from build123d import *

# Parameters (mm, degrees)
SKETCH1_R           = 6
BOSS_EXTRUDE1_DEPTH = 10
SKETCH2_R           = 1.025
CUT_EXTRUDE1_DEPTH  = 7
SKETCH4_R           = 2.1
CUT_EXTRUDE4_DEPTH  = 11.0000001
SKETCH5_W           = 0.95
SKETCH5_H           = 7.069146706
BOSS_EXTRUDE2_DEPTH = 1.2
SKETCH7_R           = 6
BOSS_EXTRUDE3_DEPTH = 1
SKETCH8_R           = 2.625
SKETCH8_W           = 2.25
SKETCH8_H           = 1.25
BOSS_EXTRUDE4_DEPTH = 6.5
SKETCH9_R           = 1.075
CUT_EXTRUDE5_DEPTH  = 6
CUT_EXTRUDE2_START  = -3
CUT_EXTRUDE2_DEPTH  = 1.85


with BuildPart() as part:
    # Sketch1 → Boss-Extrude1 (new body)
    with BuildSketch(Plane(origin=(0, 0, 0), x_dir=(1, 0, 0), z_dir=(0, 1, 0))):
        Circle(SKETCH1_R)
    extrude(amount=BOSS_EXTRUDE1_DEPTH)

    # Sketch2 → Cut-Extrude1 (cut, through all)
    with BuildSketch(Plane.XY):
        with Locations((0, 7)):
            Circle(SKETCH2_R)
    extrude(amount=-CUT_EXTRUDE1_DEPTH, mode=Mode.SUBTRACT)

    # Sketch4 → Cut-Extrude4 (cut, through all)
    with BuildSketch(Plane(origin=(0, 0, 0), x_dir=(1, 0, 0), z_dir=(0, 1, 0))):
        Circle(SKETCH4_R)
    extrude(amount=CUT_EXTRUDE4_DEPTH, mode=Mode.SUBTRACT)

    # Sketch5 → Boss-Extrude2 (add)
    with BuildSketch(Plane(origin=(0, 10, 0), x_dir=(1, 0, 0), z_dir=(0, 1, 0))):
        Rectangle(SKETCH5_W, SKETCH5_H)
    extrude(amount=-BOSS_EXTRUDE2_DEPTH)

    # Sketch7 → Boss-Extrude3 (add)
    with BuildSketch(Plane(origin=(0, 10, 0), x_dir=(1, 0, 0), z_dir=(0, 1, 0))):
        Circle(SKETCH7_R)
    extrude(amount=BOSS_EXTRUDE3_DEPTH)

    # Sketch8 → Boss-Extrude4 (add)
    with BuildSketch(Plane(origin=(0, 11, 0), x_dir=(1, 0, 0), z_dir=(0, 1, 0))):
        Circle(SKETCH8_R)
        with Locations((0, -2.625)):
            Rectangle(SKETCH8_W, SKETCH8_H)
    extrude(amount=BOSS_EXTRUDE4_DEPTH)

    # Sketch9 → Cut-Extrude5 (cut)
    with BuildSketch(Plane(origin=(0, 17.5, 0), x_dir=(1, 0, 0), z_dir=(0, 1, 0))):
        Circle(SKETCH9_R)
    extrude(amount=-CUT_EXTRUDE5_DEPTH, mode=Mode.SUBTRACT)

    # Sketch3 → Cut-Extrude2 (cut)
    with BuildSketch(Plane.XY.offset(CUT_EXTRUDE2_START)):
        Polygon((0, 4.621316891), (2.06, 5.810658445), (2.06, 8.189341555), (2.06, 11.363105915), (-2.06, 11.363105915), (-2.06, 8.189341555), (-2.06, 5.810658445), align=None)
    extrude(amount=-CUT_EXTRUDE2_DEPTH, mode=Mode.SUBTRACT)


solid = part.part
CAD build for the part. Positions are in the model's coordinates, mm. A direction names the side the tool comes from. Coordinates: 2 decimals unless noted, no trailing zeros. Write each loop counter-clockwise with the first axis right and the second up, starting at its lowest first coordinate (ties: lowest second). Pieces come first, ordered by that corner, then holes. Notation, with made-up numbers: M 56,8 L 101,8 A19 ccw 101,18 Z; hole C -37.75,25 d8. An arc over 180 degrees is marked long. Answer as a JSON object with one key per item and string values. Group by question number.
1) Saw through at D-D (y = 14). Write the cut outline in (x, z) (3 decimals), plus the area to 3 significant figures.
2) Saw through at B-B (z = 0). Write the cut outline in (x, y) (3 decimals), plus the area to 3 significant figures.
3) Saw through at A-A (y = 9.75). Write the cut outline in (x, z) (3 decimals), plus the area to 3 significant figures.
4) Wall check: line 1 (Z direction, x = 0, y = 5); line 2 (Y direction, x = 0, z = -2.75) (3 decimals); line 3 (Z direction, x = 0, y = 3.75). Give the ranges that are in metal, low to high. Write a range as from..to.
5) Pin check, flat tips, straight feed: pin 1 Ø0.7 at (y, z) = (15.5, 3) entering from +X (3 decimals); pin 2 Ø1.8 at (x, y) = (0.5, 13) entering from +Z; pin 3 Ø0.6 at (y, z) = (7.5, -4) entering from -X. Stop position of each tip, or through.
6) Saw through at C-C (x = -0.25). Write the cut outline in (y, z), plus the area to 3 significant figures.
7) Tool access for faces 5 (the face through (-0.475, 9, 0)), 6 (the face through (-1.024, 7.045, -5.418)), 7 (the face through (2.06, 8, -4)), 8 (the face through (-1.301, 5.423, 5.857)): list every direction of +Z, -Z, +X, -X, +Y, -Y with a clear straight run to the whole face (end or side of a thin tool).
8) Mould opens along X. For faces 1 (the face through (-1, 5.2, -3.9)), 2 (the face through (1.125, 14, 3)), 3 (the face through (-1, 17.5, 1)), 4 (the face through (-1.125, 14, 3)) say: +X half, -X half, draft (parallel to the pull), parting line (faces both ways), or undercut.
Values follow:
{
 "1": {"outline": "M -1.125,2.372 A2.625 ccw long 1.125,2.372 L 1.125,3.25 L -1.125,3.25 Z; hole C 0,0 d2.15", "area": "19.6 mm2"},
 "2": {"outline": "M -6,0 L -2.1,0 L -2.1,10 L -0.475,10 L -0.475,8.8 L 0.475,8.8 L 0.475,10 L 2.1,10 L 2.1,0 L 6,0 L 6,11 L 2.625,11 L 2.625,17.5 L 1.075,17.5 L 1.075,11.5 L -1.075,11.5 L -1.075,17.5 L -2.625,17.5 L -2.625,11 L -6,11 Z", "area": "112 mm2"},
 "3": {"outline": "C 0,0 d12; hole M -2.06,-4.85 L 2.06,-4.85 L 2.06,-3 L -2.06,-3 Z; hole M -0.475,-2.046 L -0.475,2.046 A2.1 ccw Z; hole M 0.475,-2.046 A2.1 ccw 0.475,2.046 Z", "area": "95.6 mm2"},
 "4": {"line 1": "z = -6..-4.85, -3..-2.1, 2.1..6", "line 2": "y = 0..5.975, 8.025..11", "line 3": "z = -6..-2.1, 2.1..6"},
 "5": {"pin 1": "stops at x = 1.125", "pin 2": "stops at z = 3.25", "pin 3": "stops at x = -4.72"},
 "6": {"outline": "M 0,-5.99 L 6.01,-5.99 L 6.01,-4.85 L 4.77,-4.85 L 4.77,-3 L 6.01,-3 L 6.01,-2.09 L 0,-2.09 Z; M 0,2.09 L 8.8,2.09 L 8.8,-2.09 L 7.99,-2.09 L 7.99,-3 L 11,-3 L 11,-2.61 L 17.5,-2.61 L 17.5,-1.05 L 11.5,-1.05 L 11.5,1.05 L 17.5,1.05 L 17.5,3.25 L 11,3.25 L 11,5.99 L 0,5.99 Z; M 7.99,-5.99 L 11,-5.99 L 11,-4.85 L 7.99,-4.85 Z", "area": "105 mm2"},
 "7": {"face 5": "-Y", "face 6": "-Z", "face 7": "+Y", "face 8": "+Y, -Y"},
 "8": {"face 1": "undercut", "face 2": "+X half", "face 3": "draft", "face 4": "-X half"}
}
